For this review, take the finished solid that the model builds, in its own axes (mm). Round coordinates to 2 decimals unless told otherwise and drop trailing zeros. Loops run counter-clockwise (first coordinate to the right, second up) from the corner with the lowest first, then second, coordinate; pieces in that order, holes last.
1. Clearance check with flat-ended pins moving along their axes: pin 1 Ø1.2 at (x, y) = (-0.5, -0.5) entering from -Z; pin 2 Ø1 at (y, z) = (0, 997.5) entering from -X; pin 3 Ø8 at (x, z) = (-6.5, 1433.5) entering from -Y. State where each tip first meets the part, or that it passes through.
2. Consider section A-A on y = -1.3. State the section outline as (x, z) points.
3. To check wall thickness, follow line 1 along X through (y, z) = (0.05, 1601); line 2 along X through (y, z) = (-0.95, 257.5); line 3 along Z through (x, y) = (-0.75, -1). State the ranges of each line that lie inside material, in increasing order.
4. Consider section B-B on z = 1494.5. State the section outline as (x, y) points, then the cut area to 3 significant figures.
from build123d import *

# Parameters (mm, degrees)
BOSS_EXTRUDE1_START = 6
SKETCH1_R           = 2
BOSS_EXTRUDE1_DEPTH = 2150
SKETCH4_R           = 2
SKETCH7_R           = 2
BOSS_EXTRUDE2_DEPTH = 2.1


with BuildPart() as part:
    # Sketch1 → Boss-Extrude1 (new body)
    with BuildSketch(Plane.XY.offset(BOSS_EXTRUDE1_START)):
        Circle(SKETCH1_R)
    extrude(amount=BOSS_EXTRUDE1_DEPTH)

    # Sketch4 → Revolve1 (revolve)
    with BuildSketch(Plane(origin=(0, 0, 0), x_dir=(-1, 0, 0), z_dir=(0, 0, -1)), mode=Mode.PRIVATE) as revolve1_sk:
        with Locations((-9, 0)):
            Circle(SKETCH4_R)
    revolve(revolve1_sk.sketch.rotate(Axis((0, 3.776003841, 0), (0, -1, 0)), 269.999990329), axis=Axis((0, 3.776003841, 0), (0, -1, 0)))

    # Sketch7 → Boss-Extrude2 (add)
    with BuildSketch(Plane(origin=(0, 0, 0), x_dir=(1, 0, 0), z_dir=(0, 1, 0))):
        with Locations(Location((0, -9, 0), (0, 0, 132.556740857))):
            Circle(SKETCH7_R)
    extrude(amount=BOSS_EXTRUDE2_DEPTH)


solid = part.part
Resolved:
1. pin 1: stops at z = -11
1. pin 2: stops at x = -2
1. pin 3: passes through
2. outline: (-1.52, 10.41) arc R10.52 ccw (long way) to (1.52, 10.41) - (1.52, 2156) - (-1.52, 2156) - close; hole (-1.52, 6) - (-1.52, 7.32) arc R7.48 ccw (long way) to (1.52, 7.32) - (1.52, 6) - close
3. line 1: x = -2 to 2
3. line 2: x = -1.76 to 1.76
3. line 3: z = -10.71 to -7.23, 6 to 2156
4. outline: circle Ø4 at (0, 0)
4. area: 12.6 mm2
